from build123d import *

# Parameters (mm, degrees)
SKETCH1_R           = 25
BOSS_EXTRUDE1_DEPTH = 10
SHELL1_T            = -1
BOSS_EXTRUDE2_DEPTH = 1
CUT_EXTRUDE1_REACH  = 94.363
SKETCH4_R           = 2.75
FILLET1_R           = 0.5
FILLET2_R           = 1.5
CUT_EXTRUDE2_REACH  = 94.363
SKETCH5_R           = 2.75


with BuildPart() as part:
    # Sketch1 → Boss-Extrude1 (new body)
    with BuildSketch(Plane(origin=(0, 0, 0), x_dir=(1, 0, 0), z_dir=(0, 1, 0))):
        with BuildLine():
            Line((13.747727085, -6), (32.078029865, 36))
            ThreePointArc((32.078029865, 36), (0, 85), (-32.078029865, 36))
            Line((-32.078029865, 36), (-13.747727085, -6))
            ThreePointArc((-13.747727085, -6), (0, -15), (13.747727085, -6))
        make_face()
        with Locations(Location((0, 50, 0), (0, 0, 270))):
            Circle(SKETCH1_R, mode=Mode.SUBTRACT)
    extrude(amount=BOSS_EXTRUDE1_DEPTH)

    # Shell1
    shell1_openings = [part.faces().sort_by_distance(p)[0] for p in [
        (-21.794129173, 10, -15.488262225),
    ]]
    offset(amount=SHELL1_T, openings=shell1_openings, kind=Kind.INTERSECTION)

    # Sketch3 → Boss-Extrude2 (add)
    with BuildSketch(Plane(origin=(0, 10, 0), x_dir=(1, 0, 0), z_dir=(0, 1, 0))):
        with BuildLine():
            Line((-23.848480035, 57.5), (23.848480035, 57.5))
            ThreePointArc((23.848480035, 57.5), (25, 50), (23.848480035, 42.5))
            Line((23.848480035, 42.5), (-23.848480035, 42.5))
            ThreePointArc((-23.848480035, 42.5), (-25, 50), (-23.848480035, 57.5))
        make_face()
    extrude(amount=-BOSS_EXTRUDE2_DEPTH)

    # Sketch4 → Cut-Extrude1 (cut, up to next)
    with BuildSketch(Plane(origin=(0, 1, 0), x_dir=(1, 0, 0), z_dir=(0, 1, 0)), mode=Mode.PRIVATE) as cut_extrude1_sk1:
        with Locations(Location((0, 0, 0), (0, 0, 270))):
            Circle(SKETCH4_R)
    cut_extrude1_tool1 = extrude(cut_extrude1_sk1.sketch, amount=-CUT_EXTRUDE1_REACH, mode=Mode.PRIVATE) & part.part
    add(cut_extrude1_tool1.solids().sort_by_distance((0, 1, 0))[0], mode=Mode.SUBTRACT)

    # Fillet1
    fillet1_edges = [part.edges().sort_by_distance(p)[0] for p in [
        (0, 1, -76),
        (0, 1, 14),
        (21.996363336, 1, -15.4),
        (0, 1, -84),
        (-21.996363336, 1, -15.4),
        (0, 1, -2.75),
    ]]
    fillet(fillet1_edges, radius=FILLET1_R)

    # Fillet2
    fillet2_edges = [part.edges().sort_by_distance(p)[0] for p in [
        (0, 0, -75),
        (-22.912878475, 0, -15),
        (0, 0, -85),
        (22.912878475, 0, -15),
        (0, 0, 15),
    ]]
    fillet(fillet2_edges, radius=FILLET2_R)

    # Sketch5 → Cut-Extrude2 (cut, up to next)
    with BuildSketch(Plane.XZ.offset(-9), mode=Mode.PRIVATE) as cut_extrude2_sk1:
        with Locations(Location((15, -50, 0), (0, 0, 270))):
            Circle(SKETCH5_R)
    cut_extrude2_tool1 = extrude(cut_extrude2_sk1.sketch, amount=-CUT_EXTRUDE2_REACH, mode=Mode.PRIVATE) & part.part
    # Sketch5 → Cut-Extrude2 (cut, up to next)
    with BuildSketch(Plane.XZ.offset(-9), mode=Mode.PRIVATE) as cut_extrude2_sk2:
        with Locations(Location((-15, -50, 0), (0, 0, 90))):
            Circle(SKETCH5_R)
    cut_extrude2_tool2 = extrude(cut_extrude2_sk2.sketch, amount=-CUT_EXTRUDE2_REACH, mode=Mode.PRIVATE) & part.part
    add(cut_extrude2_tool1.solids().sort_by_distance((15, 9, -50))[0], mode=Mode.SUBTRACT)
    add(cut_extrude2_tool2.solids().sort_by_distance((-15, 9, -50))[0], mode=Mode.SUBTRACT)


solid = part.part
CAD build for the part. Positions are in the model's coordinates, mm. A direction names the side the tool comes from. Round coordinates to 2 decimals unless told otherwise and drop trailing zeros. Loops run counter-clockwise (first coordinate to the right, second up) from the corner with the lowest first, then second, coordinate; pieces in that order, holes last. Notation, with made-up numbers: M -15.75,34.25 L 39.25,34.25 A10 cw 39.25,39.25 Z; hole C 22,-25.75 d8. An arc over 180 degrees is marked long. One line per question, with ' | ' between items. Start each with the question number.
Item 1: Cut at A-A, the plane y = 5.5. Write the cut outline in (x, z).
Item 2: Two-plate mould, pull along Z, no slides. Class faces 1 (the flat face through (22.785, 5.69, -14.706)), 2 (the cylindrical face through (-15.121, 9.493, -52.747)), 3 (the flat face through (-15, 0, -25)): pulls with the +Z half, pulls with the -Z half, needs draft (parallel to the pull), parting line crosses it, or undercut.
Item 3: Cut at B-B, the plane z = -50. State how many separate pieces and enclosed holes the cut face has, plus the area to 3 significant figures.
Item 4: Wall check: line 1 (X direction, y = 9.7, z = -50); line 2 (X direction, y = 5.25, z = -50); line 3 (Z direction, x = 22.5, y = 4.25). Give the ranges that are in metal, low to high.
Item 5: Pin check, flat tips, straight feed: pin 1 Ø1.5 at (y, z) = (4.5, -15) entering from +X; pin 2 Ø6 at (y, z) = (2, -23.5) entering from +X; pin 3 Ø1.1 at (x, y) = (5, 9.5) entering from +Z. Stop position of each tip, or through.
Item 6: Which spindle directions (+Z, -Z, +X, -X, +Y, -Y) get a long thin tool onto all of the face, cutting with end or side? Do faces 4 (the cylindrical face through (-10, 6, -26)), 5 (the cylindrical face through (0, 6, 15)), 6 (the flat face through (0, 9, -50)). Say none if no direction does.
Responses:
1) outline: M -32.08,-36 A35 ccw long 32.08,-36 L 13.75,6 A15 ccw -13.75,6 Z; C 0,-50 d52; hole M -31.16,-36.4 A34 ccw long 31.16,-36.4 L 12.83,5.6 A14 ccw -12.83,5.6 Z; hole C 0,-50 d50
2) face 1: pulls with the +Z half | face 2: undercut | face 3: needs draft
3) separate pieces: 3 | enclosed holes: 0 | area: 93.3 mm²
4) line 1: x = -35 to -34, -26 to -17.75, -12.25 to 12.25, 17.75 to 26, 34 to 35 | line 2: x = -35 to -34, -26 to -25, 25 to 26, 34 to 35 | line 3: z = -76.81 to -75.49, -63.03 to -60.9, -39.1 to -36.97, -16.55 to -14.05
5) pin 1: stops at x = 23.24 | pin 2: stops at x = 27.93 | pin 3: stops at z = 14.32
6) face 4: +Y | face 5: +Z, +Y, -Y | face 6: -Y
